from build123d import *

# Parameters (mm, degrees)
SKETCH_1_W          = 35
SKETCH_1_H          = 25
EXTRUDE_1_DEPTH     = 12
CUT_EXTRUDE_1_DEPTH = 12
SKETCH_3_W          = 35
SKETCH_3_H          = 25
CUT_EXTRUDE_2_DEPTH = 10
FILLET_1_R          = 3
FILLET_2_R          = 0.5
SKETCH_4_W          = 32
SKETCH_4_H          = 22
CUT_EXTRUDE_3_DEPTH = 10
FILLET_3_R          = 2
FILLET_4_R          = 0.5


with BuildPart() as part:
    # 草图1 → 凸台-拉伸1 (new body)
    with BuildSketch(Plane.XY):
        with Locations((-0.028271405, -3.933764136)):
            Rectangle(SKETCH_1_W, SKETCH_1_H)
    extrude(amount=EXTRUDE_1_DEPTH)

    # 草图2 → 切除-拉伸1 (cut)
    with BuildSketch(Plane(origin=(0, 0, 0), x_dir=(-1, 0, 0), z_dir=(0, 0, -1))):
        Polygon((10.837079767, 6.066235864), (5.570103523, 6.066235864), (15.028271405, 0.96567043), (15.028271405, 3.806025698), align=None)
        Polygon((0.303127279, 6.066235864), (-4.963848965, 6.066235864), (15.028271405, -4.715040108), (15.028271405, -1.874684839), align=None)
        Polygon((-10.23082521, 6.066235864), (-14.971728595, 6.066235864), (-14.971728595, 5.782537258), (15.028271405, -10.395750645), (15.028271405, -7.555395376), align=None)
        Polygon((15.028271405, -13.236105913), (-14.971728595, 2.94218199), (-14.971728595, 0.101826721), (11.054988709, -13.933764136), (15.028271405, -13.933764136), align=None)
        Polygon((5.788012464, -13.933764136), (-14.971728595, -2.738528547), (-14.971728595, -5.578883816), (0.52103622, -13.933764136), align=None)
        Polygon((-4.745940024, -13.933764136), (-14.971728595, -8.419239085), (-14.971728595, -11.259594353), (-10.012916268, -13.933764136), align=None)
    extrude(amount=-CUT_EXTRUDE_1_DEPTH, mode=Mode.SUBTRACT)

    # 草图3 → 切除-拉伸2 (cut)
    with BuildSketch(Plane.XY.offset(12)):
        with Locations((-0.028271405, -3.933764136)):
            Rectangle(SKETCH_3_W, SKETCH_3_H)
        Polygon((10.23082521, 6.066235864), (14.971728595, 6.066235864), (14.971728595, 5.782537258), (14.971728595, 2.94218199), (14.971728595, 0.101826721), (14.971728595, -2.738528547), (14.971728595, -5.578883816), (14.971728595, -8.419239085), (14.971728595, -11.259594353), (14.971728595, -13.933764136), (10.012916268, -13.933764136), (4.745940024, -13.933764136), (-0.52103622, -13.933764136), (-5.788012464, -13.933764136), (-11.054988709, -13.933764136), (-15.028271405, -13.933764136), (-15.028271405, -13.236105913), (-15.028271405, -10.395750645), (-15.028271405, -7.555395376), (-15.028271405, -4.715040108), (-15.028271405, -1.874684839), (-15.028271405, 0.96567043), (-15.028271405, 3.806025698), (-15.028271405, 6.066235864), (-10.837079767, 6.066235864), (-5.570103523, 6.066235864), (-0.303127279, 6.066235864), (4.963848965, 6.066235864), align=None, mode=Mode.SUBTRACT)
    extrude(amount=-CUT_EXTRUDE_2_DEPTH, mode=Mode.SUBTRACT)

    # 圆角1
    fillet_1_edges = [part.edges().sort_by_distance(p)[0] for p in [
        (-17.528271405, 8.566235864, 1),
        (17.471728595, 8.566235864, 1),
        (17.471728595, -16.433764136, 1),
        (-17.528271405, -16.433764136, 1),
    ]]
    fillet(fillet_1_edges, radius=FILLET_1_R)

    # 圆角2
    fillet_2_edges = [part.edges().sort_by_distance(p)[0] for p in [
        (17.471728595, -3.933764136, 0),
        (-17.528271405, -3.933764136, 0),
        (-0.028271405, 8.566235864, 0),
        (-0.028271405, -16.433764136, 0),
        (16.593048938, 7.687556208, 0),
        (-16.649591749, 7.687556208, 0),
        (-16.649591749, -15.555084479, 0),
        (16.593048938, -15.555084479, 0),
    ]]
    fillet(fillet_2_edges, radius=FILLET_2_R)

    # 草图4 → 切除-拉伸3 (cut)
    with BuildSketch(Plane.XY.offset(2)):
        with BuildLine():
            ThreePointArc((-17.528271405, -13.433764136), (-16.649591749, -15.555084479), (-14.528271405, -16.433764136))
            Line((-14.528271405, -16.433764136), (14.471728595, -16.433764136))
            ThreePointArc((14.471728595, -16.433764136), (16.593048938, -15.555084479), (17.471728595, -13.433764136))
            Line((17.471728595, -13.433764136), (17.471728595, 5.566235864))
            ThreePointArc((17.471728595, 5.566235864), (16.593048938, 7.687556208), (14.471728595, 8.566235864))
            Line((14.471728595, 8.566235864), (-14.528271405, 8.566235864))
            ThreePointArc((-14.528271405, 8.566235864), (-16.649591749, 7.687556208), (-17.528271405, 5.566235864))
            Line((-17.528271405, 5.566235864), (-17.528271405, -13.433764136))
        make_face()
        with Locations((-0.028271405, -3.933764136)):
            Rectangle(SKETCH_4_W, SKETCH_4_H, mode=Mode.SUBTRACT)
    extrude(amount=-CUT_EXTRUDE_3_DEPTH, mode=Mode.SUBTRACT)

    # 圆角3
    fillet_3_edges = [part.edges().sort_by_distance(p)[0] for p in [
        (15.971728595, 7.066235864, 1),
        (-16.028271405, 7.066235864, 1),
        (-16.028271405, -14.933764136, 1),
        (15.971728595, -14.933764136, 1),
    ]]
    fillet(fillet_3_edges, radius=FILLET_3_R)

    # 圆角4
    fillet_4_edges = [part.edges().sort_by_distance(p)[0] for p in [
        (15.971728595, -3.933764136, 0),
        (-0.028271405, 7.066235864, 0),
        (-16.028271405, -3.933764136, 0),
        (-0.028271405, -14.933764136, 0),
        (15.385942157, -14.347977698, 0),
        (-15.442484968, -14.347977698, 0),
        (-15.442484968, 6.480449427, 0),
        (15.385942157, 6.480449427, 0),
    ]]
    fillet(fillet_4_edges, radius=FILLET_4_R)


solid = part.part
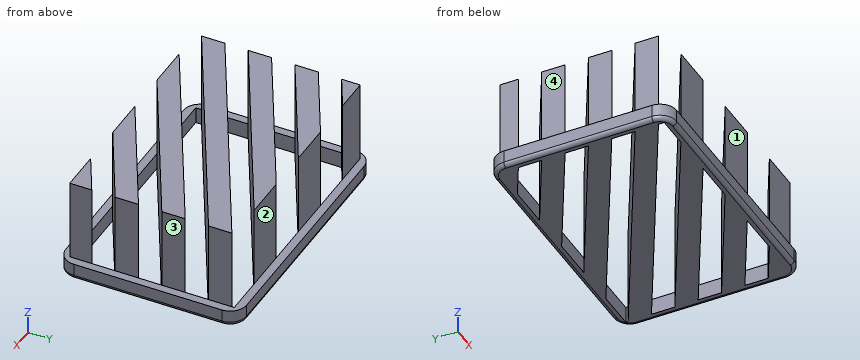
Input: part model. Units: mm. Frame: model coordinates. Face numbers are marked on the shaded views. A direction names the side the tool comes from. Coordinates: 2 decimals unless noted, no trailing zeros. Write each loop counter-clockwise with the first axis right and the second up, starting at its lowest first coordinate (ties: lowest second). Pieces come first, ordered by that corner, then holes. Notation, with made-up numbers: M 7,0 L 14,0 A28 cw 14,31 Z; hole C -38,53 d11. An arc over 180 degrees is marked long. Answer as a JSON object with one key per item and string values. Group by question number.
(1) Section B-B on x = -8.5. Output: boundary loops of the cut face in (y, z), plus the area to 3 significant figures.
(2) Section D-D on y = -0.5. Output: boundary loops of the cut face in (x, z), plus the area to 3 significant figures.
(3) Contact query for flat-ended pins moving along their axis: P1, Ø1.4, axis at y = -0.5, z = 8, coming from the +X side; P2, Ø3, axis at x = 0, y = 0.5, coming from the +Z side; P3, Ø2.5, axis at x = 6.5, z = 9.5, coming from the +Y side; P4, Ø1.4, axis at y = -11.5, z = 9, coming from the -X side. Output: stop coordinate, or through.
(4) Section A-A on z = 11.25. Output: boundary loops of the cut face in (x, y), plus the area to 3 significant figures.
(5) Set-up query: the marked faces 1, 2, 3 and 4. Return all of +Z, -Z, +X, -X, +Y, -Y with unobstructed straight access to the full face (end or side cutting, diameter ignored); none if empty.
(6) Section C-C on y = -4. Output: boundary loops of the cut face in (x, z).
(7) Ray query, line 1 along Y through (x, z) = (-6.5, 1.25); line 2 along Y through (x, z) = (-10.5, 2.5); line 3 along Y through (x, z) = (2.5, 5). Return the intervals inside material, ascending. Write a range as [from, to].
Result set:
{
 "1": {"outline": "M -14.93,0.5 A0.5 ccw -14.43,0 L -12.56,0 L -12.56,12 L -13.93,12 L -13.93,2 L -14.93,2 Z; M -9.72,0 L -6.88,0 L -6.88,12 L -9.72,12 Z; M -4.03,0 L -1.19,0 L -1.19,12 L -4.03,12 Z; M 1.65,0 L 4.49,0 L 4.49,12 L 1.65,12 Z; M 6.07,0 L 6.57,0 A0.5 ccw 7.07,0.5 L 7.07,2 L 6.07,2 Z", "area": "123 mm2"},
 "2": {"outline": "M -16.03,0.5 A0.5 ccw -15.53,0 L -12.48,0 L -12.48,12 L -15.03,12 L -15.03,2 L -16.03,2 Z; M -7.21,0 L -1.95,0 L -1.95,12 L -7.21,12 Z; M 3.32,0 L 8.59,0 L 8.59,12 L 3.32,12 Z; M 13.86,0 L 15.47,0 A0.5 ccw 15.97,0.5 L 15.97,2 L 14.97,2 L 14.97,12 L 13.86,12 Z", "area": "174 mm2"},
 "3": {"P1": "stops at x = 14.97", "P2": "stops at z = 12", "P3": "stops at y = 6.07", "P4": "stops at x = -15.03"},
 "4": {"outline": "M -15.03,-13.24 L 14.97,2.94 L 14.97,5.78 L -15.03,-10.4 Z; M -15.03,-7.56 L 10.23,6.07 L 4.96,6.07 L -15.03,-4.72 Z; M -15.03,-1.87 L -0.3,6.07 L -5.57,6.07 L -15.03,0.97 Z; M -15.03,3.81 L -10.84,6.07 L -15.03,6.07 Z; M -11.05,-13.93 L -5.79,-13.93 L 14.97,-2.74 L 14.97,0.1 Z; M -0.52,-13.93 L 4.75,-13.93 L 14.97,-8.42 L 14.97,-5.58 Z; M 10.01,-13.93 L 14.97,-13.93 L 14.97,-11.26 Z", "area": "298 mm2"},
 "5": {"face 1": "+Z, +X, -X, -Y", "face 2": "+Z, +X, -X, +Y", "face 3": "+Z, +X, +Y, -Y", "face 4": "+Z, -X, +Y, -Y"},
 "6": {"outline": "M -16.03,0.5 A0.5 ccw -15.53,0 L -15.03,0 L -15.03,2 L -16.03,2 Z; M -13.7,0 L -8.44,0 L -8.44,12 L -13.7,12 Z; M -3.17,0 L 2.1,0 L 2.1,12 L -3.17,12 Z; M 7.37,0 L 12.63,0 L 12.63,12 L 7.37,12 Z; M 14.97,0 L 15.47,0 A0.5 ccw 15.97,0.5 L 15.97,2 L 14.97,2 Z"},
 "7": {"line 1": "y = [-14.93, -11.48], [-8.64, -5.8], [-2.96, -0.12], [2.72, 5.56], [6.07, 7.07]", "line 2": "y = [-13.93, -13.63], [-10.79, -7.95], [-5.11, -2.27], [0.57, 3.41]", "line 3": "y = [-13.93, -12.3], [-9.46, -6.62], [-3.78, -0.94], [1.9, 4.74]"}
}
